Geometry: final body of the model. Coordinates: model frame, mm. Face numbers are marked on the shaded views. A direction names the side the tool comes from. Round coordinates to 2 decimals unless told otherwise and drop trailing zeros. Order: outer loops, then holes, each group sorted by start corner. A loop starts at its lowest first (then second) coordinate and runs counter-clockwise, first axis right, second up. Notation, with made-up numbers: M 31,88 L 43,88 A28 ccw 43,108 Z; hole C 16.25,76.5 d1. An arc over 180 degrees is marked long. Put each result on its own line as item: value. Start each with the question number.
1) Section A-A, the plane y = 54.5. Return loops of the section in (x, z) (3 decimals), then the cut area to 3 significant figures.
2) Section B-B, the plane z = 4. Return loops of the section in (x, y) (3 decimals), then the cut area to 3 significant figures.
3) Material intervals for probe 1 along Z at (x, y) = (41, -54) (3 decimals); probe 2 along Y at (x, z) = (60, 50.5); probe 3 along Y at (x, z) = (-29.5, 41.5), sorted ascending. Write a range as [from, to].
4) Access query for the marked faces 1, 2 and 3. Directions: +Z, -Z, +X, -X, +Y, -Y. A direction counts if a zero-diameter tool reaches every point of the face in a straight line with its end or side. Return the directions, or none.
5) First-contact query: P1, Ø12, axis at x = 44.5, z = 50.5, coming from the -Y side; P2, Ø6, axis at x = 72.5, y = -27.5, coming from the +Z side; P3, Ø5, axis at y = 20, z = 18.5, coming from the -X side (3 decimals); P4, Ø12, axis at y = -31.5, z = 34.5, coming from the -X side. Flat tips, straight axial feed; report the tip coordinate or a pass-through.
from build123d import *

# Parameters (mm, degrees)
F1_DEPTH = 63.5
F0_W     = 25.4
F0_H     = 19.05
F2_DEPTH = 25.4
F3_DEPTH = 7.9375


with BuildPart() as f1:
    # F0 (on Front) → F1 (new body, symmetric)
    with BuildSketch(Plane.XZ):
        Polygon((22.225, 9.525), (-41.275, 9.525), (-41.275, -9.525), (41.275, -9.525), (41.275, 9.525), align=None)
    extrude(amount=F1_DEPTH, both=True)

    # F0 (on Front) → F2 (join, symmetric)
    with BuildSketch(Plane.XZ):
        with BuildLine():
            Line((22.225, 27.0002), (22.225, 9.525))
            Line((22.225, 9.525), (41.275, 9.525))
            Line((41.275, 9.525), (41.275, 27.0002))
            ThreePointArc((41.275, 27.0002), (45.9246798487, 38.2255201513), (57.15, 42.8752))
            Line((57.15, 42.8752), (60.325, 42.8752))
            Line((60.325, 42.8752), (60.325, 61.9252))
            Line((60.325, 61.9252), (57.15, 61.9252))
            ThreePointArc((57.15, 61.9252), (32.4542956671, 51.6959043329), (22.225, 27.0002))
        make_face()
        with Locations((73.025, 52.4002)):
            Rectangle(F0_W, F0_H)
    extrude(amount=F2_DEPTH, both=True)

    # F0 (on Front) → F3 (join, symmetric)
    with BuildSketch(Plane.XZ):
        with BuildLine():
            add(Edge.make_bspline(
                [(-41.275, 9.525), (-40.7656654716, 59.7505532205), (9.2027997598, 62.7891719341), (57.15, 61.9252)],
                knots=[0, 0, 0, 0, 111.5045361635, 111.5045361635, 111.5045361635, 111.5045361635], degree=3))
            Line((-41.275, 9.525), (22.225, 9.525))
            Line((22.225, 9.525), (22.225, 27.0002))
            ThreePointArc((22.225, 27.0002), (32.4542956671, 51.6959043329), (57.15, 61.9252))
        make_face()
    extrude(amount=F3_DEPTH, both=True)


solid = f1.part
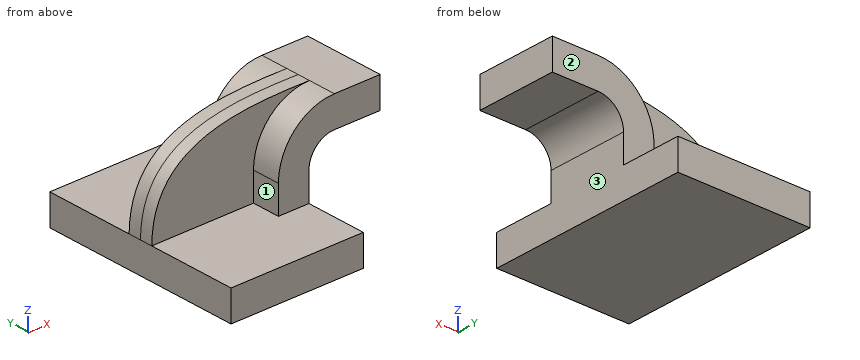
Result sheet:
1. outline: M -41.275,-9.525 L 41.275,-9.525 L 41.275,9.525 L -41.275,9.525 Z
1. area: 1,570 mm2
2. outline: M -41.275,-63.5 L 41.275,-63.5 L 41.275,63.5 L -41.275,63.5 Z
2. area: 10,500 mm2
3. probe 1: z = [-9.525, 9.525]
3. probe 2: y = [-25.4, 25.4]
3. probe 3: y = [-7.94, 7.94]
4. face 1: +Z, -X, -Y
4. face 2: +Z, +X, -X, +Y
4. face 3: -Z, +X, +Y, -Y
5. P1: stops at y = -25.4
5. P2: stops at z = 61.93
5. P3: stops at x = 22.225
5. P4: passes through
